```python
from build123d import *

# Parameters (mm, degrees)
SKETCH_R  = 1.7
PAD_DEPTH = 4


with BuildPart() as part:
    # Sketch → Pad (new body)
    with BuildSketch(Plane.XY):
        with BuildLine():
            Line((-56.499984, 48), (56.5, 48))
            ThreePointArc((59.5, 39), (61.243416, 44.581139), (56.5, 48))
            Line((59.5, 39), (59.5, -39))
            ThreePointArc((56.5, -48), (61.243416, -44.581139), (59.5, -39))
            Line((5, -48), (56.5, -48))
            Line((5, -48), (5, -36))
            ThreePointArc((5, -36), (0, -31), (-5, -36))
            Line((-5, -48), (-5, -36))
            Line((-56.5, -48), (-5, -48))
            ThreePointArc((-59.5, -39), (-61.243416, -44.581139), (-56.5, -48))
            Line((-59.5, 39), (-59.5, -39))
            ThreePointArc((-56.499984, 48), (-61.243414, 44.581147), (-59.5, 39))
        make_face()
        with Locations((-56.5, 43)):
            Circle(SKETCH_R, mode=Mode.SUBTRACT)
        with Locations((56.5, 43)):
            Circle(SKETCH_R, mode=Mode.SUBTRACT)
        with Locations((-56.5, -43)):
            Circle(SKETCH_R, mode=Mode.SUBTRACT)
        with Locations((56.5, -43)):
            Circle(SKETCH_R, mode=Mode.SUBTRACT)
    extrude(amount=PAD_DEPTH)


solid = part.part
```
Here's how the part is built. I have some questions about the finished solid (model axes, mm). A direction names the side the tool comes from. Give positions to 0.01 mm unless a question says otherwise; leave off trailing zeros. Loops run counter-clockwise (first coordinate to the right, second up) from the corner with the lowest first, then second, coordinate; pieces in that order, holes last. Notation, with made-up numbers: M 31.25,-28 L 65.25,-28 A16 cw 65.25,-3 Z; hole C 82.25,48 d6. An arc over 180 degrees is marked long. Return JSON: item names as keys, results as strings.
Item 1: I'm going to push a flat-ended pin straight in: pin 1 Ø1 at (y, z) = (-35, 3.5) entering from +X. Where does the tip first touch, or does it pass through?
A:
{"pin 1": "stops at x = 59.5"}
Item 2: Imagine slicing it at D-D on y = 23.5. List the corners of the cut face in (x, z) for me, then the cut area to 3 significant figures.
A:
{"outline": "M -59.5,0 L 59.5,0 L 59.5,4 L -59.5,4 Z", "area": "476 mm^2"}
Item 3: On a 3-axis mill with a long thin cutter (end or side, diameter ignored), from which of +Z, -Z, +X, -X, +Y, -Y can I reach the whole of each face in a straight line? I mean faces 1 (the flat face through (-59.5, 1, 2)), 2 (the flat face through (59.5, 1, 2)), 3 (the flat face through (30, -48, 2)), 4 (the flat face through (-1, 48, 2)), 5 (the flat face through (5, -42, 2)). Say none if no direction works.
A:
{"face 1": "+Z, -Z, -X", "face 2": "+Z, -Z, +X", "face 3": "+Z, -Z, +X, -X, -Y", "face 4": "+Z, -Z, +X, -X, +Y", "face 5": "+Z, -Z, -Y"}
Item 4: Imagine slicing it at B-B on z = 2.5. List the corners of the cut face in (x, y) for me, then the cut area to 3 significant figures.
A:
{"outline": "M -59.5,-39 A5 ccw -56.5,-48 L -5,-48 L -5,-36 A5 cw 5,-36 L 5,-48 L 56.5,-48 A5 ccw 59.5,-39 L 59.5,39 A5 ccw 56.5,48 L -56.5,48 A5 ccw -59.5,39 Z; hole C -56.5,-43 d3.4; hole C -56.5,43 d3.4; hole C 56.5,-43 d3.4; hole C 56.5,43 d3.4", "area": "11,300 mm^2"}
Item 5: Imagine slicing it at C-C on y = 43. List the corners of the cut face in (x, z) for me, then the cut area to 3 significant figures.
A:
{"outline": "M -61.5,0 L -58.2,0 L -58.2,4 L -61.5,4 Z; M -54.8,0 L 54.8,0 L 54.8,4 L -54.8,4 Z; M 58.2,0 L 61.5,0 L 61.5,4 L 58.2,4 Z", "area": "465 mm^2"}
Item 6: Please list where these lines run through material, in increasing order: line 1 (Y direction, x = -56.5, z = 2.2); line 2 (X direction, y = 12, z = 0.3); line 3 (X direction, y = -42.5, z = 0.4).
A:
{"line 1": "y = -48 to -44.7, -41.3 to 41.3, 44.7 to 48", "line 2": "x = -59.5 to 59.5", "line 3": "x = -61.47 to -58.12, -54.88 to -5, 5 to 54.88, 58.12 to 61.47"}
Item 7: Imagine slicing it at A-A on y = -43. List the corners of the cut face in (x, z) for me.
A:
{"outline": "M -61.5,0 L -58.2,0 L -58.2,4 L -61.5,4 Z; M -54.8,0 L -5,0 L -5,4 L -54.8,4 Z; M 5,0 L 54.8,0 L 54.8,4 L 5,4 Z; M 58.2,0 L 61.5,0 L 61.5,4 L 58.2,4 Z"}
